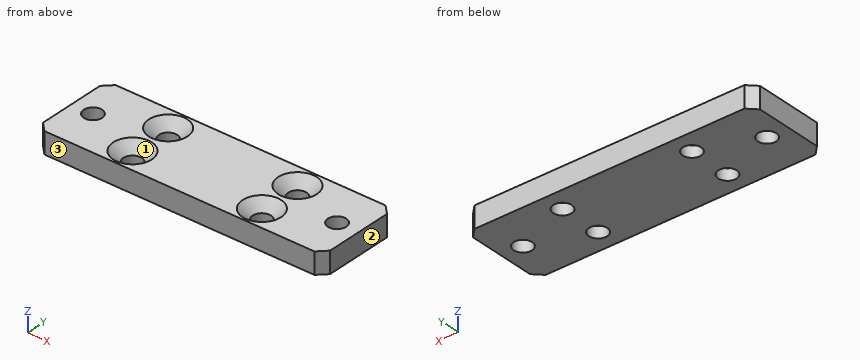
from build123d import *

# Parameters (mm, degrees)
SKETCH1_W                                            = 67
SKETCH1_H                                            = 20
BOSS_EXTRUDE1_DEPTH                                  = 2.5
M4_CLEARANCE_HOLE1_D                                 = 4.3
CSK_FOR_M4_HEX_SOCKET_COUNTERSUNK_CAP_SC_D           = 4.3
CSK_FOR_M4_HEX_SOCKET_COUNTERSUNK_CAP_SC_CSINK_D     = 9
CSK_FOR_M4_HEX_SOCKET_COUNTERSUNK_CAP_SC_CSINK_ANGLE = 90
CHAMFER1_SIZE                                        = 2


with BuildPart() as part:
    # Sketch1 → Boss-Extrude1 (new, symmetric)
    with BuildSketch(Plane.XY):
        Rectangle(SKETCH1_W, SKETCH1_H)
    extrude(amount=BOSS_EXTRUDE1_DEPTH, both=True)

    # M4 Clearance Hole1 (through all)
    with Locations(Plane.XY.offset(2.5)):
        with Locations((-28.5, 0), (28.5, 0)):
            Hole(M4_CLEARANCE_HOLE1_D / 2)

    # CSK for M4 Hex Socket Countersunk Cap Screw1 (through all)
    with Locations(Plane.XY.offset(2.5)):
        with Locations((-15.1, -5), (-15.1, 5), (15.1, 5), (15.1, -5)):
            CounterSinkHole(CSK_FOR_M4_HEX_SOCKET_COUNTERSUNK_CAP_SC_D / 2, CSK_FOR_M4_HEX_SOCKET_COUNTERSUNK_CAP_SC_CSINK_D / 2, counter_sink_angle=CSK_FOR_M4_HEX_SOCKET_COUNTERSUNK_CAP_SC_CSINK_ANGLE)

    # Chamfer1
    chamfer1_edges = [part.edges().sort_by_distance(p)[0] for p in [
        (-33.5, 10, 0),
        (33.5, 10, 0),
        (33.5, -10, 0),
        (-33.5, -10, 0),
    ]]
    chamfer(chamfer1_edges, length=CHAMFER1_SIZE)


solid = part.part
For this review, take the finished solid that the model builds, in its own axes (mm). Face numbers are marked on the shaded views. Coordinates: 2 decimals unless noted, no trailing zeros. Loops run counter-clockwise (first coordinate to the right, second up) from the corner with the lowest first, then second, coordinate; pieces in that order, holes last. Notation, with made-up numbers: (-13.75, 14) - (-8.75, 14) arc R24 cw to (-8.75, 38) - close; hole circle Ø2 at (68, -34). An arc over 180 degrees is marked (long way). Return JSON: item names as keys, results as strings.
Item 1: Take a section at A-A (x = 15.1). Give the boundary of the cut face in (y, z), then the cut area to 3 significant figures.
Determined:
{"outline": "(-10, -2.5) - (-7.15, -2.5) - (-7.15, 0.15) - (-9.5, 2.5) - (-10, 2.5) - close; (-2.85, -2.5) - (2.85, -2.5) - (2.85, 0.15) - (0.5, 2.5) - (-0.5, 2.5) - (-2.85, 0.15) - close; (7.15, -2.5) - (10, -2.5) - (10, 2.5) - (9.5, 2.5) - (7.15, 0.15) - close", "area": "46.0 mm2"}
Item 2: For line 1 (Y direction, x = -15.1, z = -1.05); line 2 (X direction, y = -5, z = -0.75); line 3 (X direction, y = -4, z = -1.8), list the stretches that pass through material, from the lowest coordinate up.
Determined:
{"line 1": "y = -10 to -7.15, -2.85 to 2.85, 7.15 to 10", "line 2": "x = -33.5 to -17.25, -12.95 to 12.95, 17.25 to 33.5", "line 3": "x = -33.5 to -17, -13.2 to 13.2, 17 to 33.5"}
Item 3: Take a section at B-B (y = 5). Give the boundary of the cut face in (x, z).
Determined:
{"outline": "(-33.5, -2.5) - (-17.25, -2.5) - (-17.25, 0.15) - (-19.6, 2.5) - (-33.5, 2.5) - close; (-12.95, -2.5) - (12.95, -2.5) - (12.95, 0.15) - (10.6, 2.5) - (-10.6, 2.5) - (-12.95, 0.15) - close; (17.25, -2.5) - (33.5, -2.5) - (33.5, 2.5) - (19.6, 2.5) - (17.25, 0.15) - close"}
Item 4: Take a section at D-D (x = 27). Give the boundary of the cut face in (y, z), then the cut area to 3 significant figures.
Determined:
{"outline": "(-10, -2.5) - (-1.54, -2.5) - (-1.54, 2.5) - (-10, 2.5) - close; (1.54, -2.5) - (10, -2.5) - (10, 2.5) - (1.54, 2.5) - close", "area": "84.6 mm2"}
Item 5: Take a section at C-C (x = -28.5). Give the boundary of the cut face in (y, z).
Determined:
{"outline": "(-10, -2.5) - (-2.15, -2.5) - (-2.15, 2.5) - (-10, 2.5) - close; (2.15, -2.5) - (10, -2.5) - (10, 2.5) - (2.15, 2.5) - close"}
Item 6: Insertion check: pin 1 (5.5 mm diameter, centred on x = 15.1, y = -5, fed in from -Z). The pin has a flat end and moves straight along its axis. Give the tip position at first contact, or say it passes through.
Determined:
{"pin 1": "stops at z = -2.5"}
Item 7: Mouldability with a two-part tool opening along X and no side actions: class the marked faces 1, 2 and 3 as pulls with the +X half, pulls with the -X half, needs draft (parallel to the pull), parting line crosses it, or undercut.
Determined:
{"face 1": "undercut", "face 2": "pulls with the +X half", "face 3": "needs draft"}
